```python
from build123d import *

# Parameters (mm, degrees)
F1_DEPTH = 1.57
F2_DEPTH = 3.14
F4_DEPTH = 0.5
F5_DEPTH = 3.14
F6_DEPTH = 0.785


with BuildPart() as f1:
    # F0 (on Front) → F1 (new body)
    with BuildSketch(Plane.XZ):
        with BuildLine():
            ThreePointArc((0, 1.4), (0.9899494937, 0.9899494937), (1.4, 0))
            ThreePointArc((1.4, 0), (1.0722010752, -0.9002137826), (0.2423073508, -1.3788716937))
            Line((0.2423073508, -1.3788716937), (5.03, -1.3788716937))
            ThreePointArc((5.03, -1.3788716937), (4.6072316639, 0), (5.03, 1.3788716937))
            Line((5.03, 1.3788716937), (5.03, 1.4))
            Line((5.03, 1.4), (0, 1.4))
        make_face()
    extrude(amount=F1_DEPTH)

    # F0 (on Front) → F2 (join)
    with BuildSketch(Plane.XZ):
        with BuildLine():
            ThreePointArc((5.03, 1.3788716937), (4.6072316639, 0), (5.03, -1.3788716937))
            ThreePointArc((5.03, -1.3788716937), (7.1531686939, -2.4584984903), (9.1957705087, -1.2332568208))
            Line((9.1957705087, -1.2332568208), (7.9895535242, -1.2332568208))
            ThreePointArc((7.9895535242, -1.2332568208), (5.5273609556, -0.0199549945), (7.9572859214, 1.2567431792))
            Line((7.9572859214, 1.2567431792), (9.1819885249, 1.2567431792))
            ThreePointArc((9.1819885249, 1.2567431792), (7.139559961, 2.458936481), (5.03, 1.3788716937))
        make_face()
    extrude(amount=F2_DEPTH)

    # F3 (on face) → F4 (cut)
    with BuildSketch(Plane(origin=(0, 0, 0), x_dir=(-1, 0, 0), z_dir=(0, 1, 0))):
        with BuildLine():
            ThreePointArc((-5.03, 1.4), (-4.8076942376, 0.0105641531), (-5.03, -1.3788716937))
            Line((-5.03, -1.3788716937), (-0.2423073508, -1.3788716937))
            ThreePointArc((-0.2423073508, -1.3788716937), (-1.3947079213, 0.1216133808), (0, 1.4))
            Line((0, 1.4), (-5.03, 1.4))
        make_face()
    extrude(amount=-F4_DEPTH, mode=Mode.SUBTRACT)

    # F0 (on Front) → F5 (join)
    with BuildSketch(Plane.XZ):
        with BuildLine():
            ThreePointArc((0.2423073508, -1.3788716937), (1.0722010752, -0.9002137826), (1.4, 0))
            ThreePointArc((1.4, 0), (0.9899494937, 0.9899494937), (0, 1.4))
            ThreePointArc((0, 1.4), (-1.3947079213, -0.1216133808), (0.2423073508, -1.3788716937))
        make_face()
    extrude(amount=F5_DEPTH)

    # F6 (add): a face of the model
    f6_faces = [f1.faces().sort_by_distance(p)[0] for p in [
        (2.9154968292, -1.57, 0.0141355812),
    ]]
    extrude(f6_faces, amount=F6_DEPTH)


solid = f1.part
```
Part model, mm, in its own coordinate system. A direction names the side the tool comes from. Give positions to 0.01 mm unless a question says otherwise; leave off trailing zeros. Loops run counter-clockwise (first coordinate to the right, second up) from the corner with the lowest first, then second, coordinate; pieces in that order, holes last. Notation, with made-up numbers: M 30,-39 L 53,-39 A21 cw 53,-19 Z; hole C -4,-24 d9. An arc over 180 degrees is marked long. Return JSON: item names as keys, results as strings.
1) 3-axis set-ups, long thin cutter, end or side, ignore diameter. For faces 3 (the face through (0, 0, 0)), 4 (the face through (3, -1, 1.4)), 5 (the face through (9, -2, -1.233)), 6 (the face through (3, -1, -1.379)): which of +Z, -Z, +X, -X, +Y, -Y reach the whole face in a straight line?
Calculated:
{"face 3": "+Z, -Z, +X, -X, +Y", "face 4": "+Z, -X, +Y, -Y", "face 5": "+X, +Y, -Y", "face 6": "-Z, +Y, -Y"}
2) Saw through at C-C, the plane y = -2.9. List the corners of the cut face in (x, z).
Calculated:
{"outline": "C 0,0 d2.8; M 7.96,1.26 L 9.18,1.26 A2.46 ccw long 9.2,-1.23 L 7.99,-1.23 A1.54 cw long Z"}
3) Saw through at B-B, the plane x = 6.75. List the corners of the cut face in (y, z).
Calculated:
{"outline": "M -3.14,-2.44 L 0,-2.44 L 0,-1.51 L -3.14,-1.51 Z; M -3.14,1.51 L 0,1.51 L 0,2.44 L -3.14,2.44 Z"}
4) Flat gauge pins, fed straight in: pin 1 Ø1 at (x, y) = (0.5, -2) entering from +Z; pin 2 Ø0.6 at (x, y) = (8.5, -1.5) entering from +Z; pin 3 Ø0.9 at (x, y) = (3, -2) entering from -Z. Where does each tip first touch, or does it go through?
Calculated:
{"pin 1": "stops at z = 1.4", "pin 2": "stops at z = 2.18", "pin 3": "stops at z = -1.38"}
5) Pull direction X, two halves, no side cores. Call faces 1 (the face through (5, -3.14, 0)), 2 (the face through (5.53, -1.55, -0.07)): released by +X, released by -X, zero draft, split by the parting line, or undercut.
Calculated:
{"face 1": "zero draft", "face 2": "undercut"}
6) Drill centre lines: line 1 (Z direction, x = 2, y = -1.8); line 2 (Y direction, x = 1.75, z = 1.1) (3 decimals); line 3 (X direction, y = -0.95, z = 0). Where is each one in solid material? Low to high.
Calculated:
{"line 1": "z = -1.38 to 1.4", "line 2": "y = -2.355 to -0.5", "line 3": "x = -1.4 to 5.53"}
